Can you work these out from the model? Positions are in its coordinate system, mm. A direction names the side the tool comes from. Give positions to 0.01 mm unless a question says otherwise; leave off trailing zeros. Write each loop counter-clockwise with the first axis right and the second up, starting at its lowest first coordinate (ties: lowest second). Pieces come first, ordered by that corner, then holes. Notation, with made-up numbers: (-11.5, 71) -> (41.5, 71) arc R13 cw to (41.5, 93) -> close; hole circle Ø3 at (-5.75, 10.5). An arc over 180 degrees is marked (long way). One line per item, written item: value.
from build123d import *

# Parameters (mm, degrees)
F1_E0_W  = 12.2108995656
F1_E0_H  = 25.4
F2_DEPTH = 1.5875
F1_E1_W  = 5.4040532559
F1_E1_H  = 25.4
F1_E2_W  = 12.6289542233
F1_E2_H  = 25.4
F3_DEPTH = 1.5875
F5_DEPTH = 6.35
F7_DEPTH = 25.4
F9_DEPTH = 3.683


with BuildPart() as f2:
    # F1_E0 (on explicit) → F2 (new body)
    with BuildSketch(Plane(origin=(-11.4085562527, 0, 0), x_dir=(0.6884263284, 0, 0.7253062735), z_dir=(0.7253062735, 0, -0.6884263284))):
        with Locations((6.1054497828, 12.7)):
            Rectangle(F1_E0_W, F1_E0_H)
    extrude(amount=F2_DEPTH)

    # F1_E1 (on explicit) + F1_E2 (on explicit) → F3 (join)
    with BuildSketch(Plane(origin=(-3.0022514984, 0, 8.85664206), x_dir=(1, 0, 0), z_dir=(0, 0, -1))):
        with Locations((2.702026628, 12.7)):
            Rectangle(F1_E1_W, F1_E1_H)
    with BuildSketch(Plane(origin=(2.4018017575, 0, 8.85664206), x_dir=(0.7128696552, 0, -0.7012965526), z_dir=(-0.7012965526, 0, -0.7128696552))):
        with Locations((6.3144771116, 12.7)):
            Rectangle(F1_E2_W, F1_E2_H)
    extrude(amount=F3_DEPTH, dir=(0, 0, -1))

    # F4 (on face) → F5 (cut)
    with BuildSketch(Plane(origin=(-4.850266242, 0, 4.6036427682), x_dir=(0, 1, 0), z_dir=(0.7253062735, 0, -0.6884263284))):
        Polygon((0, 3.6749982582), (-25.4, -7.8539504933), (0, -7.8539504933), align=None)
    extrude(amount=-F5_DEPTH, mode=Mode.SUBTRACT)

    # F6 (on face) → F7 (cut)
    with BuildSketch(Plane(origin=(4.8153308136, 0, 4.8947955096), x_dir=(0.7128696552, 0, -0.7012965526), z_dir=(-0.7012965526, 0, -0.7128696552))):
        Polygon((9.2433015468, 25.4), (-3.3856526765, 0), (9.2433015468, 0), align=None)
    extrude(amount=-F7_DEPTH, mode=Mode.SUBTRACT)

    # F8 (on face) → F9 (cut)
    with BuildSketch(Plane(origin=(0, 0, 8.85664206), x_dir=(1, 0, 0), z_dir=(0, 0, -1))):
        Polygon((0.017724813, 21.7312984169), (-0.0206197838, 21.7312984169), (-0.0206197838, 0), (0.0242347851, 0), align=None)
    extrude(amount=F9_DEPTH, mode=Mode.SUBTRACT)


solid = f2.part
1) For faces 1 (the face through (5.84, -15.7, 5.474)), 2 (the face through (-4.58, -18.52, 4.89)), which set-ups out of +Z, -Z, +X, -X, +Y, -Y let a thin tool reach every point of the face, with its end or its side?
Answer list:
face 1: +Z, +X, +Y, -Y
face 2: -Z, +Y, -Y
2) We'd pull the mould along X, two halves only. Please class faces 3 (the face through (7.36, -12.88, 3.18)), 4 (the face through (5.84, -15.7, 3.887)), 5 (the face through (-0.3, -12.9, 8.857)): released by +X, released by -X, zero draft, split by the parting line, or undercut.
Answer list:
face 3: released by +X
face 4: undercut
face 5: zero draft
3) Will these pins go through, and if not, where does the flat tip stop? pin 1 (1.5 mm diameter, centred on y = -12, z = 5.5, fed in from -X); pin 2 (1.3 mm diameter, centred on y = -8.5, z = 7.5, fed in from +X); pin 3 (3 mm diameter, centred on y = -11.5, z = 2.5, fed in from -X); pin 4 (1 mm diameter, centred on y = -9, z = 2.5, fed in from -X).
Answer list:
pin 1: stops at x = -6.9
pin 2: stops at x = 4.44
pin 3: stops at x = -6.74
pin 4: passes through
4) If we section it at B-B (y = -11.25): Write out the boundary of the cut face in (x, z).
Answer list:
outline: (-6.99, 4.66) -> (-5.84, 3.57) -> (-2.32, 7.27) -> (-0.02, 7.27) -> (-0.02, 8.86) -> (-3, 8.86) -> close; (0.02, 7.27) -> (2.4, 7.27) -> (6.39, 3.35) -> (7.18, 4.15) -> (2.4, 8.86) -> (0.02, 8.86) -> close
5) If we section it at A-A (z = 6.25): Write out the boundary of the cut face in (x, y).
Answer list:
outline: (-5.48, -25.4) -> (-3.29, -25.4) -> (-3.29, -3.1) -> (-5.48, -6.42) -> close; (3.44, -25.4) -> (5.05, -25.4) -> (5.05, -5.24) -> (3.44, -2.92) -> close
6) I need wall thicknesses on L1, parallel to X at y = -23, z = 6.5; L2, parallel to X at y = -15, z = 2.5; L3, parallel to X at y = -22.5, z = -0.25. Which ranges of each line are inside material? Lowest first, please.
Answer list:
L1: x = -5.24 to -3.05, 3.18 to 4.8
L2: x = -7.19 to -6.85, 7.25 to 8.17
L3: x = 10.05 to 10.7
7) If we section it at C-C (z = 1.5): Write out the boundary of the cut face in (x, y).
Answer list:
outline: (-9.98, -25.4) -> (-7.8, -25.4) -> (-7.8, -17.52) -> (-9.98, -20.84) -> close; (8.27, -25.4) -> (9.88, -25.4) -> (9.88, -18.86) -> (8.27, -16.55) -> close
